Answer from the drawing. Dimensions are ordinates in mm from the lowest x, y and z of the part. A direction names the side the tool comes from. Coordinates: 2 decimals unless noted, no trailing zeros. Write each loop counter-clockwise with the first axis right and the second up, starting at its lowest first coordinate (ties: lowest second). Pieces come first, ordered by that corner, then holes. Notation, with made-up numbers: (35.25, 82) -> (73.25, 82) arc R13 ccw to (73.25, 88) -> close; hole circle Ø2 at (27, 16.25). An arc over 180 degrees is marked (long way). Answer as a JSON object with one key per item and string values. Group by question number.
(1) Find section C-C (x = 20). Give the vertices of the cut face in (y, z).
(2) Find section B-B (y = 10.5). Give the vertices of the cut face in (x, z).
(3) Flat-ended cylindrical pins translate along their axes: P1, Ø7, axis at x = 20, z = 25, coming from the -Y side; P2, Ø1.6, axis at x = 1, y = 11, coming from the +Z side. Find the tip coordinate at first contact, or state that the pin passes through.
(4) Which of the six approach directions +Z, -Z, +X, -X, +Y, -Y give full straight-line access (tool end or side, diameter ignored) to the marked faces 1 and 2?
(5) Straight lines are drawn through the part: L1, parallel to Z at x = 20, y = 6.25; L2, parallel to X at y = 21.5, z = 25; L3, parallel to X at y = 5, z = 25. For each, find the intervals that lie inside material, in ascending order.
(6) Find section A-A (z = 105). Give the vertices of the cut face in (x, y), then the cut area to 3 significant figures.
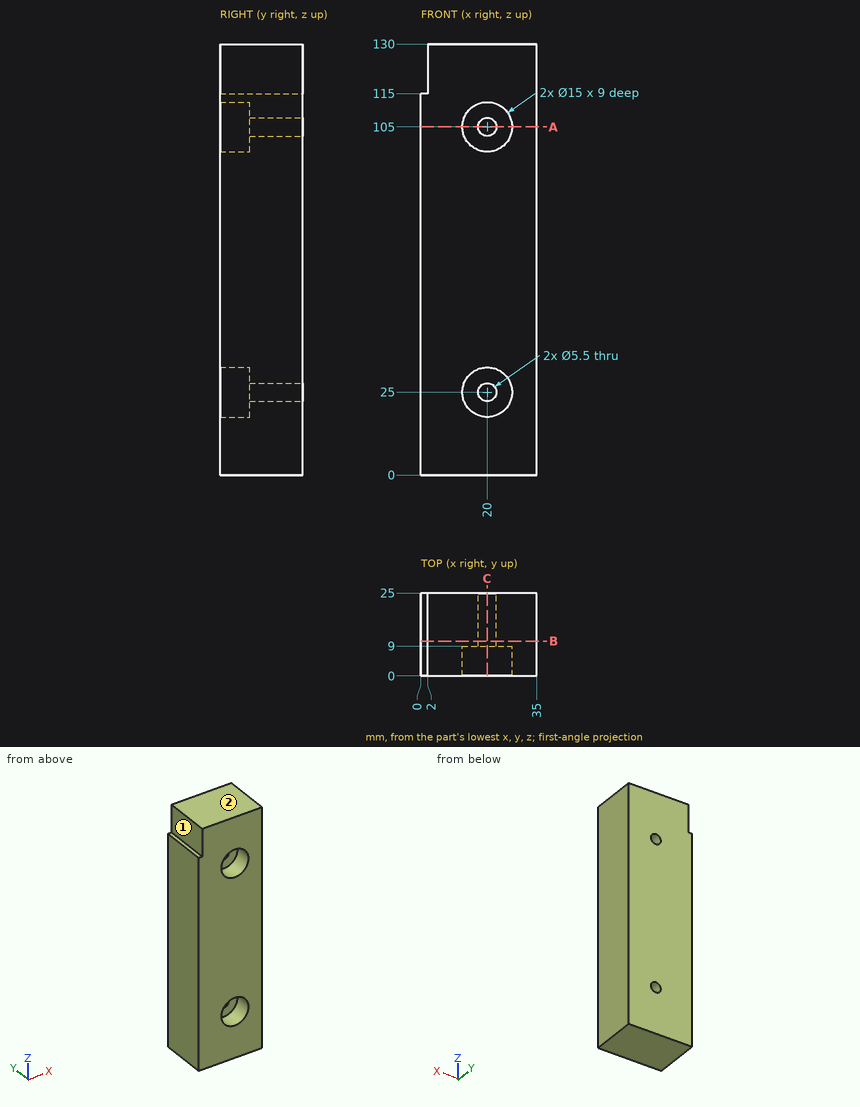
Results below:
{
 "1": {"outline": "(0, 0) -> (25, 0) -> (25, 22.25) -> (9, 22.25) -> (9, 17.5) -> (0, 17.5) -> close; (0, 32.5) -> (9, 32.5) -> (9, 27.75) -> (25, 27.75) -> (25, 102.25) -> (9, 102.25) -> (9, 97.5) -> (0, 97.5) -> close; (0, 112.5) -> (9, 112.5) -> (9, 107.75) -> (25, 107.75) -> (25, 130) -> (0, 130) -> close"},
 "2": {"outline": "(0, 0) -> (35, 0) -> (35, 130) -> (2, 130) -> (2, 115) -> (0, 115) -> close; hole circle Ø5.5 at (20, 25); hole circle Ø5.5 at (20, 105)"},
 "3": {"P1": "stops at y = 9", "P2": "stops at z = 115"},
 "4": {"face 1": "+Z, -X, +Y, -Y", "face 2": "+Z, +X, -X, +Y, -Y"},
 "5": {"L1": "z = 0 to 17.5, 32.5 to 97.5, 112.5 to 130", "L2": "x = 0 to 17.25, 22.75 to 35", "L3": "x = 0 to 12.5, 27.5 to 35"},
 "6": {"outline": "(0, 0) -> (12.5, 0) -> (12.5, 9) -> (17.25, 9) -> (17.25, 25) -> (0, 25) -> close; (22.75, 9) -> (27.5, 9) -> (27.5, 0) -> (35, 0) -> (35, 25) -> (22.75, 25) -> close", "area": "652 mm2"}
}
